Autodesk Fusion 360 part; units mm, degrees
sketch "Sketch1" plane through (0, 0, 0) normal (0, 0, 1) x (1, 0, 0)
  line L0 (0, 0) -> (80, 0)
  line L1 (80, 0) -> (80, 80)
  line L2 (80, 80) -> (0, 80)
  line L3 (0, 80) -> (0, 0)
  circle A0 centre (40, 68.5) radius 1.5
  circle A1 centre (40, 11.5) radius 1.5
  dimension "d1" = 80
  dimension "d2" = 80
  dimension "d3" = 3
  dimension "d4" = 3
  dimension "d5" = 57
  dimension "d6" = 40
  dimension "d7" = 40
  dimension "d8" = 11.5
extrude "Extrude1" add sketch "Sketch1" along normal blind 2.5
Work out the finished part from the listing and answer in its coordinate system (mm). Coordinates: 2 decimals unless noted, no trailing zeros. Order: outer loops, then holes, each group sorted by start corner. A loop starts at its lowest first (then second) coordinate and runs counter-clockwise, first axis right, second up. Notation, with made-up numbers: M 80.25,-6.5 L 125.25,-6.5 A18 ccw 125.25,17.5 Z; hole C 46,58 d6. An arc over 180 degrees is marked long. Use CSV: the item, a comma, the result in double quotes.
1) A flat-ended cylindrical pin translates along its axis: pin 1 Ø2 at (x, y) = (47, 66.5) entering from -Z. Find the tip coordinate at first contact, or state that the pin passes through.
Worked out:
pin 1,"stops at z = 0"
2) Determine the mould class of faces 1 (the face through (0, 41, 1)), 2 (the face through (39, 41, 0)), 3 (the face through (38.8, 12.4, 1.2)), 4 (the face through (80, 39, 1)) for opening direction X: released by +X, released by -X, zero draft, split by the parting line, or undercut.
Worked out:
face 1,"released by -X"
face 2,"zero draft"
face 3,"undercut"
face 4,"released by +X"
3) Consider line 1 (Y direction, x = 40, z = 0.9); line 2 (X direction, y = 68.5, z = 0.75). Determine where each line is inside the solid, lowest interval first. Write a range as [from, to].
Worked out:
line 1,"y = [0, 10], [13, 67], [70, 80]"
line 2,"x = [0, 38.5], [41.5, 80]"
4) Section B-B on y = 11.5 is taken. Write down the section's boundary in (x, z).
Worked out:
outline,"M 0,0 L 38.5,0 L 38.5,2.5 L 0,2.5 Z; M 41.5,0 L 80,0 L 80,2.5 L 41.5,2.5 Z"
5) Section A-A on x = 40 is taken. Write down the section's boundary in (y, z).
Worked out:
outline,"M 0,0 L 10,0 L 10,2.5 L 0,2.5 Z; M 13,0 L 67,0 L 67,2.5 L 13,2.5 Z; M 70,0 L 80,0 L 80,2.5 L 70,2.5 Z"
